```python
from build123d import *

# Parameters (mm, degrees)
ESBO_O1_R                  = 12.5
RESSALTO_EXTRUS_O1_DEPTH   = 4.064
ESBO_O2_R                  = 12.5
ESBO_O2_R_2                = 10
RESSALTO_EXTRUS_O2_DEPTH   = 15
CORTE_EXTRUS_O1_DEPTH      = 24
CORTE_EXTRUS_O1_DEPTH_BACK = 23
ESBO_O3_R                  = 2.5


with BuildPart() as part:
    # Esboço1 → Ressalto-extrusão1 (new body)
    with BuildSketch(Plane.XY):
        Circle(ESBO_O1_R)
    extrude(amount=RESSALTO_EXTRUS_O1_DEPTH)

    # Esboço2 → Ressalto-extrusão2 (add)
    with BuildSketch(Plane.XY.offset(4.064)):
        Circle(ESBO_O2_R)
        Circle(ESBO_O2_R_2, mode=Mode.SUBTRACT)
    extrude(amount=RESSALTO_EXTRUS_O2_DEPTH)

    # Esboço3 → Corte-extrusão1 (cut, two sides: drawn at the far end of the back side and taken through both)
    with BuildSketch(Plane(origin=(0, 0, 0), x_dir=(0, 0, -1), z_dir=(1, 0, 0)).offset(-CORTE_EXTRUS_O1_DEPTH_BACK)):
        with Locations(Location((-14.564, 0, 0), (0, 0, 180))):
            Circle(ESBO_O3_R)
        with Locations(Location((-4.564, 0, 0), (0, 0, 180))):
            Circle(ESBO_O3_R)
    extrude(amount=CORTE_EXTRUS_O1_DEPTH + CORTE_EXTRUS_O1_DEPTH_BACK, mode=Mode.SUBTRACT)


solid = part.part
```
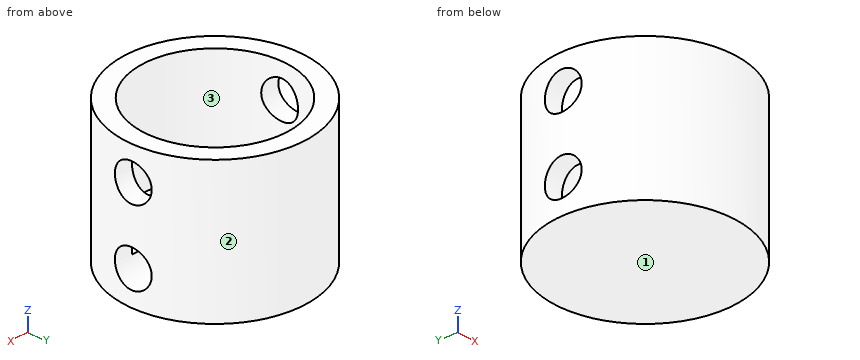
Check sheet for the modelled part. Datum: model origin and axes. Units: mm. Face numbers are marked on the shaded views. Round coordinates to 2 decimals unless told otherwise and drop trailing zeros. Write each loop counter-clockwise with the first axis right and the second up, starting at its lowest first coordinate (ties: lowest second). Pieces come first, ordered by that corner, then holes. Notation, with made-up numbers: M -5.5,-20 L 41.5,-20 A19 ccw 41.5,8 Z; hole C -27,66 d5. An arc over 180 degrees is marked long. Write item = value, one per line. Start each with the question number.
1. Gauge pin test, flat ends, axial feed: pin 1 (1.5 mm diameter, centred on y = 6, z = 12, fed in from +X); pin 2 (4 mm diameter, centred on y = 3.5, z = 14.5, fed in from +X); pin 3 (1.5 mm diameter, centred on x = -9, z = 11.5, fed in from -Y); pin 4 (4.5 mm diameter, centred on y = 0, z = 14.564, fed in from -X). Record the tip position at first contact, or that the pin passes through.
2. Release check for a two-part mould opening along X. For the marked faces 1, 2 and 3 record: pulls with the +X half, pulls with the -X half, needs draft (parallel to the pull), parting line crosses it, or undercut.
3. Section check D-D, the plane x = 11. Record the cut outline in (y, z).
4. Section check C-C, the plane x = 0. Record the cut outline in (y, z), then the cut area to 3 significant figures.
5. Section check B-B, the plane z = 6.25. Record the cut outline in (x, y).
6. Scan lines: line 1 (Y direction, x = 0, z = 9); line 2 (Z direction, x = -1, y = -9.25); line 3 (Y direction, x = 5.25, z = 6). Record each from-to range of solid material in increasing order. Write a range as [from, to].
7. Section check A-A, the plane y = 0. Record the cut outline in (x, z).
Results found:
q1.pin_1 = 11.34
q1.pin_2 = 12.33
q1.pin_3 = -9.39
q1.pin_4 = through
q2.face_1 = needs draft
q2.face_2 = parting line crosses it
q2.face_3 = undercut
q3.outline = M -5.94,0 L 5.94,0 L 5.94,19.06 L -5.94,19.06 Z; hole C 0,4.56 d5; hole C 0,14.56 d5
q4.outline = M -12.5,0 L 12.5,0 L 12.5,19.06 L 10,19.06 L 10,4.06 L 2.45,4.06 A2.5 cw -2.45,4.06 L -10,4.06 L -10,19.06 L -12.5,19.06 Z
q4.area = 169 mm^2
q5.outline = M -12.36,-1.85 A12.5 ccw 12.36,-1.85 L 9.83,-1.85 A10 cw -9.83,-1.85 Z; M -12.36,1.85 L -9.83,1.85 A10 cw 9.83,1.85 L 12.36,1.85 A12.5 ccw Z
q6.line_1 = [-12.5, -10], [10, 12.5]
q6.line_2 = [0, 4.06]
q6.line_3 = [-11.34, -8.51], [8.51, 11.34]
q7.outline = M -12.5,0 L 12.5,0 L 12.5,2.06 L -12.5,2.06 Z; M -12.5,7.06 L -10,7.06 L -10,12.06 L -12.5,12.06 Z; M -12.5,17.06 L -10,17.06 L -10,19.06 L -12.5,19.06 Z; M 10,7.06 L 12.5,7.06 L 12.5,12.06 L 10,12.06 Z; M 10,17.06 L 12.5,17.06 L 12.5,19.06 L 10,19.06 Z
